For this review, take the finished solid that the model builds, in its own axes (mm). Face numbers are marked on the shaded views. A direction names the side the tool comes from. Give positions to 0.01 mm unless a question says otherwise; leave off trailing zeros. Write each loop counter-clockwise with the first axis right and the second up, starting at its lowest first coordinate (ties: lowest second). Pieces come first, ordered by that corner, then holes. Notation, with made-up numbers: M 83.5,69 L 133.5,69 A16 ccw 133.5,77 Z; hole C -1.75,42.25 d10. An arc over 180 degrees is marked long. Write item = value, one per line.
```python
from build123d import *

# Parameters (mm, degrees)
BOSS_EXTRUDE1_DEPTH = 3.175


with BuildPart() as part:
    # Sketch1 → Boss-Extrude1 (new body)
    with BuildSketch(Plane.XY):
        with BuildLine():
            Line((-27.95, 18.625), (-1.95, 18.625))
            Line((-1.95, 18.625), (-1.95, 5.963704675))
            Line((-1.95, 5.963704675), (-4.95, 5.963704675))
            Line((-4.95, 5.963704675), (-4.95, 3.353294588))
            Line((-4.95, 3.353294588), (-1.95, 3.353294588))
            Line((-1.95, 3.353294588), (-1.95, 2.795))
            Line((-1.95, 2.795), (-1.95, -0.255))
            ThreePointArc((-1.95, -0.255), (-2.535786438, -1.669213562), (-3.95, -2.255))
            Line((-3.95, -2.255), (-25.95, -2.255))
            ThreePointArc((-25.95, -2.255), (-27.364213562, -1.669213562), (-27.95, -0.255))
            Line((-27.95, -0.255), (-27.95, 2.795))
            Line((-27.95, 2.795), (-27.95, 3.353294588))
            Line((-27.95, 3.353294588), (-24.95, 3.353294588))
            Line((-24.95, 3.353294588), (-24.95, 5.963704675))
            Line((-24.95, 5.963704675), (-27.95, 5.963704675))
            Line((-27.95, 5.963704675), (-27.95, 18.625))
        make_face()
    extrude(amount=BOSS_EXTRUDE1_DEPTH)


solid = part.part
```
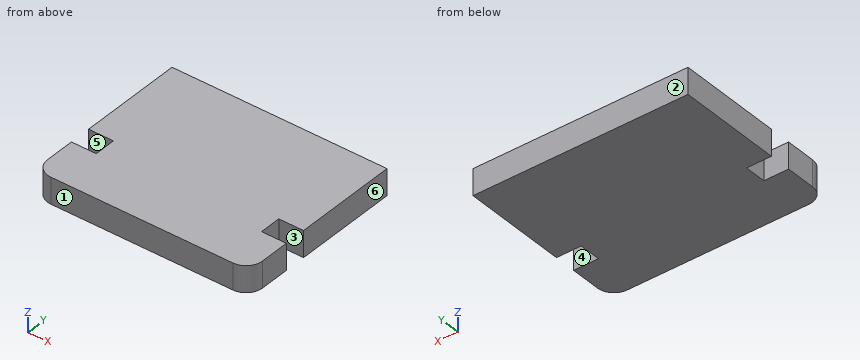
1. We need section A-A, the plane z = 1.75. Write out the cut boundary in (x, y) (3 decimals), then the cut area to 4 significant figures.
Responses:
outline = M -27.95,-0.255 A2 ccw -25.95,-2.255 L -3.95,-2.255 A2 ccw -1.95,-0.255 L -1.95,3.353 L -4.95,3.353 L -4.95,5.964 L -1.95,5.964 L -1.95,18.625 L -27.95,18.625 L -27.95,5.964 L -24.95,5.964 L -24.95,3.353 L -27.95,3.353 Z
area = 525.5 mm2
2. We need section B-B, the plane y = 4.75. Write out the cut boundary in (x, z) (3 decimals).
Responses:
outline = M -24.95,0 L -4.95,0 L -4.95,3.175 L -24.95,3.175 Z
3. Insertion check: P1, Ø0.9, axis at x = -3.5, z = 1, coming from the -Y side (3 decimals). The pin has a flat end and moves straight along its axis. Give the tip position at first contact, or say it passes through.
Responses:
P1 = -2.255
4. For line 1 along Y through (x, z) = (-4.75, 2.55) (3 decimals); line 2 along X through (y, z) = (5.5, 0.65); line 3 along Y through (x, z) = (-3.75, 0.4) (3 decimals), list the stretches that pass through material, from the lowest coordinate up. Write a range as from..to.
Responses:
line_1 = -2.255..3.353, 5.964..18.625
line_2 = -24.95..-4.95
line_3 = -2.245..3.353, 5.964..18.625
5. The part is to be moulded in two halves that separate along Y. For the marked faces 1, 2 and 3, say which applies: +Y half, -Y half, draft (parallel to the pull), parting line (faces both ways), or undercut.
Responses:
face_1 = -Y half
face_2 = +Y half
face_3 = undercut
6. Machinability: for the marked faces 4, 5 and 6, which of the approach directions +Z, -Z, +X, -X, +Y, -Y give a long, thin tool a straight path to every point of the face, cutting with its end or side? Answer none if there is none.
Responses:
face_4 = +Z, -Z, +X
face_5 = +Z, -Z, -X
face_6 = +Z, -Z, +X, +Y, -Y
